Could you check a few things on this drawing? It's one solid part, dimensions in mm from its lowest x, y, z. A direction names the side the tool comes from. Give positions to 0.01 mm unless a question says otherwise; leave off trailing zeros. Loops run counter-clockwise (first coordinate to the right, second up) from the corner with the lowest first, then second, coordinate; pieces in that order, holes last.
1. For P1, Ø12, axis at x = 5.5, z = 17, coming from the +Y side; P2, Ø1, axis at x = 3, y = 3, coming from the +Z side; P3, Ø1, axis at x = 16, z = 8.5, coming from the +Y side, each with a flat end and sliding along its axis, tell me the tip position at first contact or that it passes through.
2. I need wall thicknesses on line 1 along X through (y, z) = (3.65, 10); line 2 along Y through (x, z) = (10, 1.7); line 3 along Y through (x, z) = (16, 17). Which ranges of each line are inside material? Lowest first, please.
3. Imagine slicing it at A-A (z = 10). List the corners of the cut face in (x, y) for me.
4. Thinking about a two-plate mould opening in Y: for the marked faces 3, 4 and 5, which applies, +Y half, -Y half, draft (parallel to the pull), parting line (faces both ways), or undercut?
5. Imagine slicing it at D-D (y = 2.75). List the corners of the cut face in (x, z) for me.
6. Imagine slicing it at C-C (x = 10). List the corners of the cut face in (y, z) for me.
7. For the marked faces 1 and 2, which set-ups out of +Z, -Z, +X, -X, +Y, -Y let a thin tool reach every point of the face, with its end or its side?
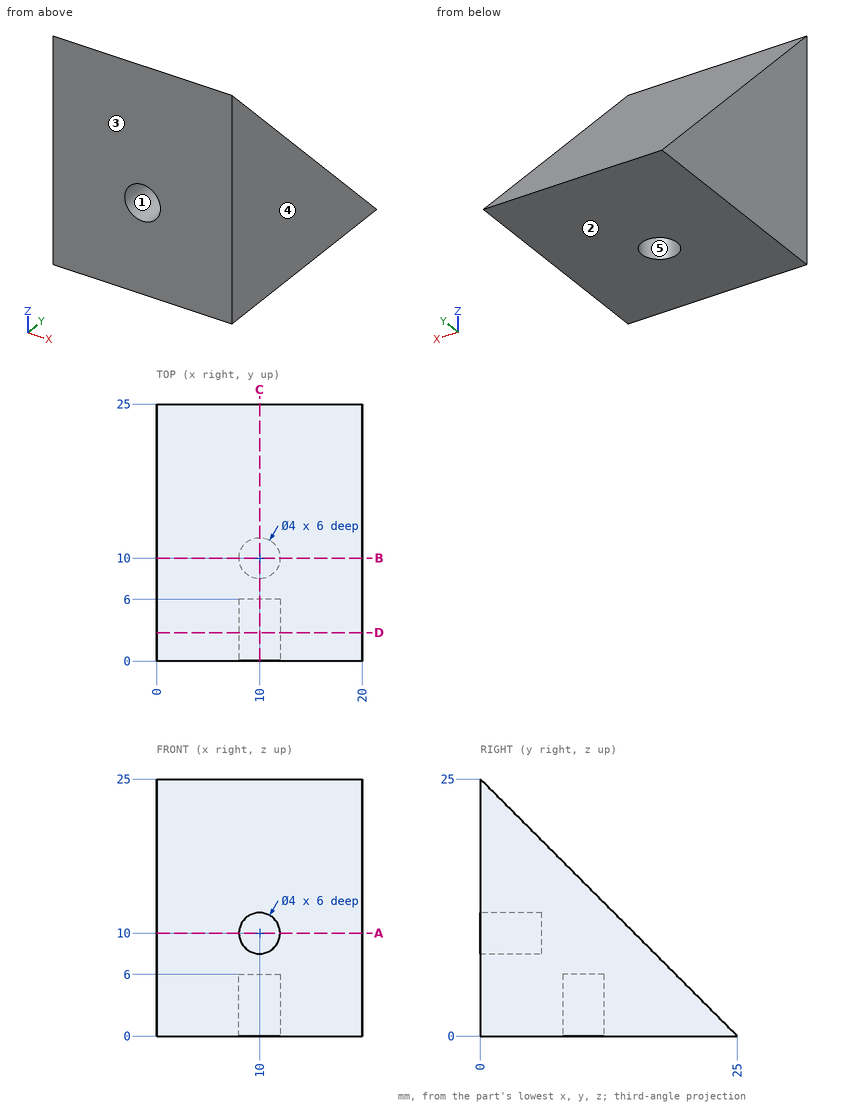
Derived:
1. P1: stops at y = 14
1. P2: stops at z = 22.5
1. P3: stops at y = 17
2. line 1: x = 0 to 8, 12 to 20
2. line 2: y = 0 to 8, 12 to 23.3
2. line 3: y = 0 to 8
3. outline: (0, 0) - (8, 0) - (8, 6) - (12, 6) - (12, 0) - (20, 0) - (20, 15) - (0, 15) - close
4. face 3: -Y half
4. face 4: draft
4. face 5: undercut
5. outline: (0, 0) - (20, 0) - (20, 22.25) - (0, 22.25) - close; hole circle Ø4 at (10, 10)
6. outline: (0, 0) - (8, 0) - (8, 6) - (12, 6) - (12, 0) - (25, 0) - (0, 25) - (0, 12) - (6, 12) - (6, 8) - (0, 8) - close
7. face 1: -Y
7. face 2: -Z, +X, -X, +Y, -Y
